Check sheet for the drawn part. Datum: minimum x, y, z corner. Units: mm. Give positions to 0.01 mm unless a question says otherwise; leave off trailing zeros. Loops run counter-clockwise (first coordinate to the right, second up) from the corner with the lowest first, then second, coordinate; pieces in that order, holes last. Notation, with made-up numbers: M 19,74 L 57,74 A14 cw 57,88 Z; hole C -5,88.25 d6. An arc over 180 degrees is marked long. Write each question's results on one line, items separated by ' | '. Start each with the question number.
1. Sectioned sample at B-B on y = 4.75. Record the cut outline in (x, z).
2. Material ranges on line 1 along Y through (x, z) = (23, 0.3); line 2 along X through (y, z) = (6.5, 0.6); line 3 along Z through (x, y) = (17, 22), recorded low to high.
3. Go/stop test with flat-tipped pins: pin 1 (14.5 mm diameter, centred on x = 20, y = 14, fed in from -Z); pin 2 (0.8 mm diameter, centred on x = 21, z = 0.5, fed in from +Y); pin 3 (0.5 mm diameter, centred on x = 17, z = 0.5, fed in from -Y). Record where each tip stops, or that it passes through.
4. Sectioned sample at C-C on x = 43. Record the cut outline in (y, z).
5. Draft check along Y on the marked faces 1 and 2. Enter one of: pulls with the +Y half, pulls with the -Y half, needs draft (parallel to the pull), parting line crosses it, or undercut.
6. Sectioned sample at A-A on z = 0.3. Record the cut outline in (x, y).
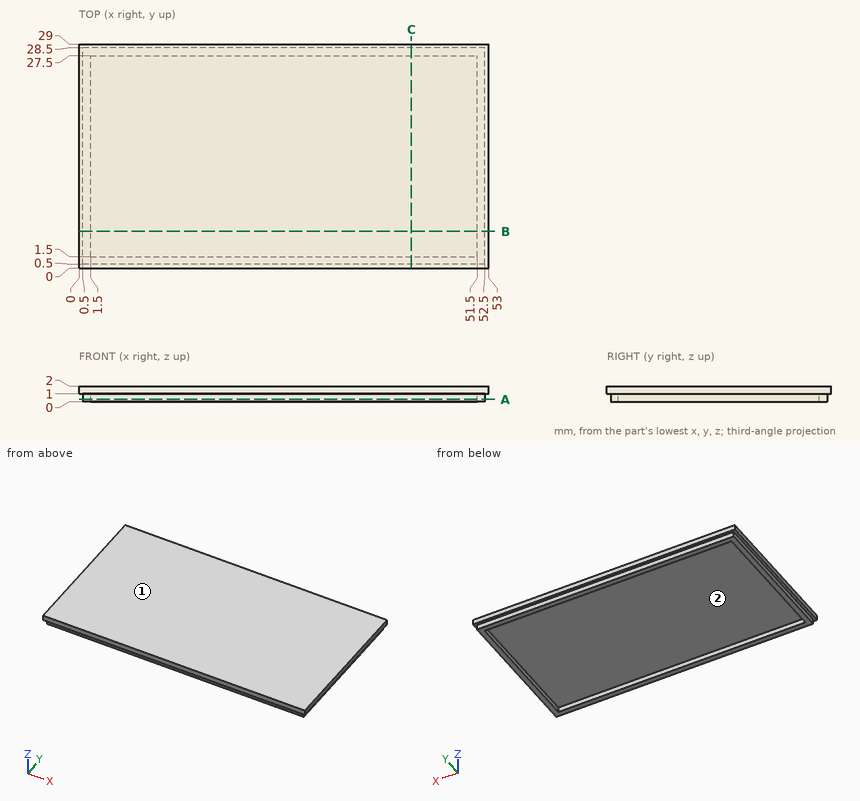
Output values:
1) outline: M 0,1 L 0.5,1 L 0.5,0 L 1.5,0 L 1.5,1 L 51.5,1 L 51.5,0 L 52.5,0 L 52.5,1 L 53,1 L 53,2 L 0,2 Z
2) line 1: 0.5 to 1.5, 27.5 to 28.5 | line 2: 0.5 to 1.5, 51.5 to 52.5 | line 3: 1 to 2
3) pin 1: z = 1 | pin 2: y = 28.5 | pin 3: y = 0.5
4) outline: M 0,1 L 0.5,1 L 0.5,0 L 1.5,0 L 1.5,1 L 27.5,1 L 27.5,0 L 28.5,0 L 28.5,1 L 29,1 L 29,2 L 0,2 Z
5) face 1: needs draft | face 2: undercut
6) outline: M 0.5,0.5 L 52.5,0.5 L 52.5,28.5 L 0.5,28.5 Z; hole M 1.5,1.5 L 51.5,1.5 L 51.5,27.5 L 1.5,27.5 Z
